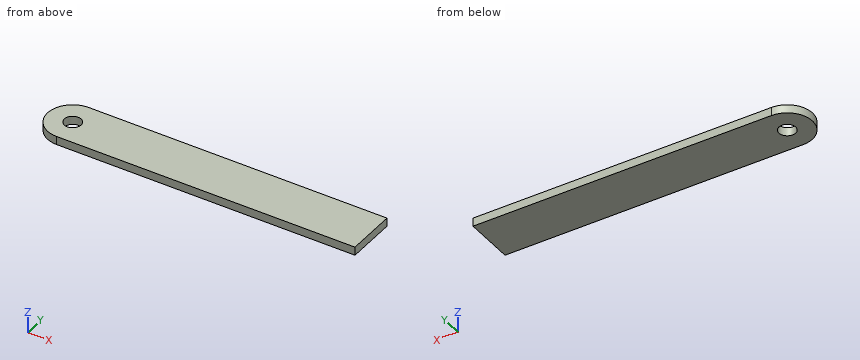
```python
from build123d import *

# Parameters (mm, degrees)
ESQUISSE1_R                  = 2
BOSS_EXTRU_1_DEPTH           = 2
ENL_V_MAT_EXTRU_1_DEPTH      = 78.757636281
ENL_V_MAT_EXTRU_1_DEPTH_BACK = 78.757636281


with BuildPart() as part:
    # Esquisse1 → Boss.-Extru.1 (new body)
    with BuildSketch(Plane.XY):
        with BuildLine():
            Line((-71.5, 6), (71.5, 6))
            ThreePointArc((71.5, 6), (77.5, 0), (71.5, -6))
            Line((71.5, -6), (-71.5, -6))
            ThreePointArc((-71.5, -6), (-77.5, 0), (-71.5, 6))
        make_face()
        with Locations((-71.5, 0)):
            Circle(ESQUISSE1_R, mode=Mode.SUBTRACT)
        with Locations((71.5, 0)):
            Circle(ESQUISSE1_R, mode=Mode.SUBTRACT)
    extrude(amount=BOSS_EXTRU_1_DEPTH)

    # Esquisse3 → Enlèv. mat.-Extru.1 (cut, two sides: drawn at the far end of the back side and taken through both)
    with BuildSketch(Plane.XY.offset(2).offset(-ENL_V_MAT_EXTRU_1_DEPTH_BACK)):
        Polygon((0, 0), (0, 10.962701513), (80.234264698, 10.962701513), (80.234264698, -13.981416423), (0, -13.981416423), align=None)
    extrude(amount=ENL_V_MAT_EXTRU_1_DEPTH + ENL_V_MAT_EXTRU_1_DEPTH_BACK, mode=Mode.SUBTRACT)


solid = part.part
```
For this review, take the finished solid that the model builds, in its own axes (mm). Round coordinates to 2 decimals unless told otherwise and drop trailing zeros. Write each loop counter-clockwise with the first axis right and the second up, starting at its lowest first coordinate (ties: lowest second). Pieces come first, ordered by that corner, then holes. Notation, with made-up numbers: M 74,40.5 L 87,40.5 A20 cw 87,78.5 Z; hole C 62,43.25 d2. An arc over 180 degrees is marked long. One line per item, written item: value. Start each with the question number.
(1) We need section B-B (z = 0.5). Give the boundary of the cut face in (x, y).
(2) We need section C-C (y = 3.75). Give the boundary of the cut face in (x, z).
(3) We need section A-A (y = 0). Give the boundary of the cut face in (x, z).
(4) Wall thickness on line 1 (Y direction, x = -71.5, z = 1.4); line 2 (X direction, y = 0.5, z = 1.05); line 3 (X direction, y = 1, z = 1.6): over which ranges is each line inside the solid? List them lowest first.
Result:
1. outline: M -71.5,-6 L 0,-6 L 0,6 L -71.5,6 A6 ccw Z; hole C -71.5,0 d4
2. outline: M -76.18,0 L 0,0 L 0,2 L -76.18,2 Z
3. outline: M -77.5,0 L -73.5,0 L -73.5,2 L -77.5,2 Z; M -69.5,0 L 0,0 L 0,2 L -69.5,2 Z
4. line 1: -6 to -2, 2 to 6
4. line 2: -77.48 to -73.44, -69.56 to 0
4. line 3: -77.42 to -73.23, -69.77 to 0
